from build123d import *

# Parameters (mm, degrees)
ESBO_O1_W                = 25
ESBO_O1_H                = 10
ESBO_O1_R                = 4.05
RESSALTO_EXTRUS_O1_DEPTH = 10
RESSALTO_EXTRUS_O2_DEPTH = 10
RESSALTO_EXTRUS_O3_REACH = 32.394
ESBO_O3_W                = 1.752399307
ESBO_O3_H                = 1.5


with BuildPart() as part:
    # Esboço1 → Ressalto-extrusão1 (new body)
    with BuildSketch(Plane(origin=(0, 0, 0), x_dir=(1, 0, 0), z_dir=(0, 1, 0))):
        Rectangle(ESBO_O1_W, ESBO_O1_H)
        with Locations(Location((0, 0, 0), (0, 0, 270))):
            Circle(ESBO_O1_R, mode=Mode.SUBTRACT)
    extrude(amount=RESSALTO_EXTRUS_O1_DEPTH)

    # Esboço2 → Ressalto-extrusão2 (add)
    with BuildSketch(Plane.XZ):
        Polygon((-12.5, 5), (-12.5, 11.7), (-10.1, 14.1), (10.1, 14.1), (12.5, 11.7), (12.5, 5), (10.1, 5), (10.1, 11.7), (-10.1, 11.7), (-10.1, 5), align=None)
    extrude(amount=-RESSALTO_EXTRUS_O2_DEPTH)

    # Esboço3 → Ressalto-extrusão3 (add, up to next)
    with BuildSketch(Plane.ZY.offset(12.5), mode=Mode.PRIVATE) as ressalto_extrus_o3_sk1:
        with Locations((5.154994999, 9.25)):
            Rectangle(ESBO_O3_W, ESBO_O3_H)
    ressalto_extrus_o3_tool1 = extrude(ressalto_extrus_o3_sk1.sketch, amount=-RESSALTO_EXTRUS_O3_REACH, mode=Mode.PRIVATE) - part.part
    add(ressalto_extrus_o3_tool1.solids().sort_by_distance((-12.5, 9.25, 5.154995))[0])


solid = part.part
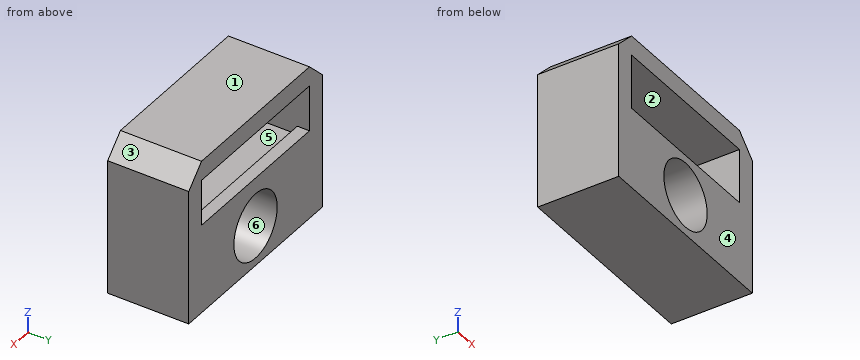
CAD build for the part. Positions are in the model's coordinates, mm. Face numbers are marked on the shaded views. A direction names the side the tool comes from. Round coordinates to 2 decimals unless told otherwise and drop trailing zeros. Write each loop counter-clockwise with the first axis right and the second up, starting at its lowest first coordinate (ties: lowest second). Pieces come first, ordered by that corner, then holes.
(1) Slice it at B-B, the plane x = 0. Write the cut outline in (y, z).
(2) Probe line 1 along X through (y, z) = (4.5, 0); line 2 along X through (y, z) = (1.75, 6); line 3 along Z through (x, y) = (-7.25, 1.5). List the from-to ranges inside material, lowest first.
(3) Slice it at D-D, the plane y = 4. Write the cut outline in (x, z), and give its area (3 significant figures).
(4) Slice it at A-A, the plane z = 8. Write the cut outline in (x, y).
(5) Slice it at C-C, the plane x = -4.5. Write the cut outline in (y, z), and give its area (3 significant figures).
(6) 3-axis set-ups, long thin cutter, end or side, ignore diameter. For the marked faces 1 and 2: which of +Z, -Z, +X, -X, +Y, -Y reach the whole face in a straight line?
(7) Mould opens along X. For the marked faces 3, 4, 5 and 6 say: pulls with the +X half, pulls with the -X half, needs draft (parallel to the pull), parting line crosses it, or undercut.
From the geometry:
1. outline: (0, -5) - (10, -5) - (10, -4.05) - (0, -4.05) - close; (0, 4.05) - (10, 4.05) - (10, 6.03) - (8.5, 6.03) - (8.5, 5) - (0, 5) - close; (0, 11.7) - (10, 11.7) - (10, 14.1) - (0, 14.1) - close
2. line 1: x = -12.5 to -4.05, 4.05 to 12.5
2. line 2: x = -12.5 to -10.1, 10.1 to 12.5
2. line 3: z = -5 to 5, 11.7 to 14.1
3. outline: (-12.5, -5) - (12.5, -5) - (12.5, 11.7) - (10.1, 14.1) - (-10.1, 14.1) - (-12.5, 11.7) - close; hole (-10.1, 5) - (10.1, 5) - (10.1, 11.7) - (-10.1, 11.7) - close; hole circle Ø8.1 at (0, 0)
3. area: 285 mm2
4. outline: (-12.5, 0) - (-10.1, 0) - (-10.1, 10) - (-12.5, 10) - close; (10.1, 0) - (12.5, 0) - (12.5, 10) - (10.1, 10) - close
5. outline: (0, -5) - (10, -5) - (10, 6.03) - (8.5, 6.03) - (8.5, 5) - (0, 5) - close; (0, 11.7) - (10, 11.7) - (10, 14.1) - (0, 14.1) - close
5. area: 126 mm2
6. face 1: +Z, +X, -X, +Y, -Y
6. face 2: +Y, -Y
7. face 3: pulls with the +X half
7. face 4: needs draft
7. face 5: undercut
7. face 6: undercut
